```python
from build123d import *

# Parameters (mm, degrees)
SKETCH2_R           = 12
SKETCH2_R_2         = 3.2639
BOSS_EXTRUDE1_DEPTH = 3.175
BOSS_EXTRUDE2_DEPTH = 3.175
CIRPATTERN1_COUNT   = 8


with BuildPart() as part:
    # Sketch2 → Boss-Extrude1 (new body)
    with BuildSketch(Plane(origin=(0, 0, 0), x_dir=(-1, 0, 0), z_dir=(0, 1, 0))):
        with Locations(Location((0, 0, 0), (0, 0, 90))):
            Circle(SKETCH2_R)
        with Locations(Location((0, 0, 0), (0, 0, 90))):
            Circle(SKETCH2_R_2, mode=Mode.SUBTRACT)
    extrude(amount=BOSS_EXTRUDE1_DEPTH)

    # Sketch2_3 → Boss-Extrude2 (add)
    with BuildSketch(Plane(origin=(0, 0, 0), x_dir=(-1, 0, 0), z_dir=(0, 1, 0))):
        with BuildLine():
            ThreePointArc((-1.660095527, 11.884615385), (0, 12), (1.660095527, 11.884615385))
            ThreePointArc((1.660095527, 11.884615385), (1.210599357, 12.066020943), (0.899218411, 12.4375))
            ThreePointArc((0.899218411, 12.4375), (0, 13), (-0.899218411, 12.4375))
            ThreePointArc((-0.899218411, 12.4375), (-1.210599357, 12.066020943), (-1.660095527, 11.884615385))
        make_face()
    boss_extrude2 = extrude(amount=BOSS_EXTRUDE2_DEPTH)

    # CirPattern1: Boss-Extrude2 ×8 about axis
    cirpattern1_axis = Axis((0, 0, 0), (0, 1, 0))
    for i in range(1, CIRPATTERN1_COUNT):
        add(boss_extrude2.rotate(cirpattern1_axis, i * 360 / CIRPATTERN1_COUNT))


solid = part.part
```
Design review of the part built by this model. Coordinates are the model's own, in mm. Coordinates: 2 decimals unless noted, no trailing zeros. Order: outer loops, then holes, each group sorted by start corner. A loop starts at its lowest first (then second) coordinate and runs counter-clockwise, first axis right, second up. Notation, with made-up numbers: (27, 27.25) - (48, 27.25) arc R17 cw to (48, 36.25) - close; hole circle Ø4 at (-4, -34). An arc over 180 degrees is marked (long way). Answer in a Markdown table with one row per item.
(1) Consider section A-A on x = 0. State the section outline as (y, z) points (3 decimals).
Checked values:
| item | result |
|---|---|
| outline | (0, -13) - (3.175, -13) - (3.175, -3.264) - (0, -3.264) - close; (0, 3.264) - (3.175, 3.264) - (3.175, 13) - (0, 13) - close |
(2) The part is to be moulded in two halves that separate along X. For faces 1 (the flat face through (-3, 3.175, -3)), 2 (the cylindrical face through (4.553, 1.565, 11.103)), 3 (the cylindrical face through (-11.103, 1.565, 4.553)), 4 (the cylindrical face through (-3.186, 1.565, -0.708)), say which applies: released by +X, released by -X, zero draft, split by the parting line, or undercut.
Checked values:
| item | result |
|---|---|
| face 1 | zero draft |
| face 2 | released by +X |
| face 3 | released by -X |
| face 4 | undercut |
(3) Wall thickness on line 1 along X through (y, z) = (1.65, 0); line 2 along Z through (x, y) = (2, 0.4); line 3 along Z through (x, y) = (-1.75, 2.65): over which ranges is each line inside the solid? List them lowest first. Write a range as from..to.
Checked values:
| item | result |
|---|---|
| line 1 | -13..-3.26, 3.26..13 |
| line 2 | -11.83..-2.58, 2.58..11.83 |
| line 3 | -11.87..-2.76, 2.76..11.87 |
(4) Consider section D-D on x = 4. State the section outline as (y, z) points (3 decimals), plus the area to 3 significant figures.
Checked values:
| item | result |
|---|---|
| outline | (0, -11.314) - (3.175, -11.314) - (3.175, 11.314) - (0, 11.314) - close |
| area | 71.8 mm^2 |
(5) Clearance check with a flat-ended pin moving along its axis: pin 1 (6 mm diameter, centred on x = 0, z = 0, fed in from +Y) (1 decimal). State where the tip first meets the part, or that it passes through.
Checked values:
| item | result |
|---|---|
| pin 1 | through |
(6) Consider section B-B on z = 0. State the section outline as (x, y) points (3 decimals), plus the area to 3 significant figures.
Checked values:
| item | result |
|---|---|
| outline | (-13, 0) - (-3.264, 0) - (-3.264, 3.175) - (-13, 3.175) - close; (3.264, 0) - (13, 0) - (13, 3.175) - (3.264, 3.175) - close |
| area | 61.8 mm^2 |
